from build123d import *
from build123d.topology import SkipClean

# Parameters (mm, degrees)
SKETCH2_R               = 70.00000000000001
BOSS_EXTRUDE1_DEPTH     = 500
SKETCH5_R               = 70.00000000000003
CUT_EXTRUDE1_DEPTH      = 500
CUT_EXTRUDE2_DEPTH      = 70
CUT_EXTRUDE2_DEPTH_BACK = 100
SKETCH6_W               = 70
SKETCH6_H               = 140
CUT_EXTRUDE3_DEPTH      = 120
CUT_EXTRUDE3_DEPTH_BACK = 100
SKETCH7_R               = 25
SKETCH8_R               = 25.000000000000007
CUT_EXTRUDE4_DEPTH      = 50


with BuildPart() as part:
    # Sketch2 → Boss-Extrude1 (new body)
    with BuildSketch(Plane(origin=(0, 0, 0), x_dir=(1, 0, 0), z_dir=(0, 1, 0))):
        with Locations(Location((0, 0, 0), (0, 0, 270))):
            Circle(SKETCH2_R)
    extrude(amount=BOSS_EXTRUDE1_DEPTH)

    # Sketch3 one side → Revolve1 (revolve)
    with SkipClean():  # the faces are left unmerged after this step: merging them gives an invalid solid
        with BuildSketch(Plane(origin=(0, 0, 0), x_dir=(-1, 0, 0), z_dir=(0, -1, 0))):
            with BuildLine():
                ThreePointArc((-1.505e-12, -70.00000000000001), (49.497474683057796, -49.49747468305888), (70.00000000000001, -2.07e-14))
                ThreePointArc((70.00000000000001, -3.55e-15), (49.497474683058854, 49.49747468305782), (1.46534e-12, 70.00000000000001))
                Line((0, 70.00000000000001), (0, -70.00000000000001))
            make_face()
        revolve(axis=Axis((0, 0, 0), (0, 0, 1)))

    # Sketch4 → Revolve2 (revolve)
    with SkipClean():  # the faces are left unmerged after this step: merging them gives an invalid solid
        with BuildSketch(Plane(origin=(0, 500, 0), x_dir=(1, 0, 0), z_dir=(0, 1, 0))):
            with BuildLine():
                Line((0, 70.00000000000001), (0, -70.00000000000001))
                ThreePointArc((0, -70.00000000000001), (70.00000000000001, 0), (0, 70.00000000000001))
            make_face()
        revolve(axis=Axis((0, 500, -70.00000000000001), (0, 0, 1)))

    # Sketch5 → Cut-Extrude1 (cut)
    with SkipClean():  # the faces are left unmerged after this step: merging them gives an invalid solid
        with BuildSketch(Plane(origin=(0, 0, 0), x_dir=(0, 0, -1), z_dir=(1, 0, 0))):
            with Locations((0, 500)):
                Circle(SKETCH5_R)
        extrude(amount=-CUT_EXTRUDE1_DEPTH, mode=Mode.SUBTRACT)

    # Sketch6 → Cut-Extrude2 (cut, two sides: drawn at the far end of the back side and taken through both)
    with BuildSketch(Plane(origin=(0, 0, 0), x_dir=(1, 0, 0), z_dir=(0, 1, 0)).offset(-CUT_EXTRUDE2_DEPTH_BACK)):
        Rectangle(SKETCH6_W, SKETCH6_H)
    extrude(amount=CUT_EXTRUDE2_DEPTH + CUT_EXTRUDE2_DEPTH_BACK, mode=Mode.SUBTRACT)

    # Sketch7 → Cut-Extrude3 (cut, two sides: drawn at the far end of the back side and taken through both)
    with BuildSketch(Plane.ZY.offset(-35).offset(-CUT_EXTRUDE3_DEPTH_BACK)):
        with Locations(Location((0, 0, 0), (0, 0, 180))):
            Circle(SKETCH7_R)
    extrude(amount=CUT_EXTRUDE3_DEPTH + CUT_EXTRUDE3_DEPTH_BACK, mode=Mode.SUBTRACT)

    # Sketch8 → Cut-Extrude4 (cut)
    with BuildSketch(Plane.ZY):
        with Locations((0, 500)):
            Circle(SKETCH8_R)
    extrude(amount=-CUT_EXTRUDE4_DEPTH, mode=Mode.SUBTRACT)


solid = part.part
For this review, take the finished solid that the model builds, in its own axes (mm). A direction names the side the tool comes from. Round coordinates to 2 decimals unless told otherwise and drop trailing zeros. Order: outer loops, then holes, each group sorted by start corner. A loop starts at its lowest first (then second) coordinate and runs counter-clockwise, first axis right, second up. Notation, with made-up numbers: M 12,88 L 71,88 A15 cw 71,117 Z; hole C -26.5,86.25 d9. An arc over 180 degrees is marked long. Write each question's results on one line, items separated by ' | '. Start each with the question number.
1. Clearance check with flat-ended pins moving along their axes: pin 1 Ø12 at (x, z) = (-17.5, -26.5) entering from -Y; pin 2 Ø5 at (x, z) = (52.5, -3.5) entering from -Y; pin 3 Ø1.5 at (x, y) = (43.5, 211.5) entering from +Z. State where each tip first meets the part, or that it passes through.
2. Add section B-B (x = 25). State the section outline as (y, z) points, then the cut area to 3 significant figures.
3. To check wall thickness, follow L1, parallel to Y at x = -57, z = 11.5; L2, parallel to X at y = 246, z = -4; L3, parallel to Z at x = 43, y = -10.5. State the ranges of each line that lie inside material, in increasing order. Write a range as [from, to].
4. Draft analysis for pull direction Z (two halves, no side actions). For faces 5 (the face through (35, 33, 1)), 6 (the face through (52.7, 22.2, -11.5)), 7 (the face through (69.404, 246.5, -9.113)), state which applies: pulls with the +Z half, pulls with the -Z half, needs draft (parallel to the pull), parting line crosses it, or undercut.
5. Add section A-A (z = 0). State the section outline as (x, y) points, then the cut area to 3 significant figures.
6. Tool access review of faces 1 (the face through (24.65, 524.787, -3.255)), 2 (the face through (-52.3, 22.2, -11.5)), 3 (the face through (-26.732, 430.017, 1.539)), 4 (the face through (0, 70, -1)): name each direction out of +Z, -Z, +X, -X, +Y, -Y from which nothing blocks a thin tool from reaching the whole face with its end or side.
7. Add section D-D (y = 104.5). State the section outline as (x, z) points, then the cut area to 3 significant figures.
8. Add section C-C (z = 36.5). State the section outline as (x, y) points.
Output values:
1) pin 1: y = 70 | pin 2: y = -48.87 | pin 3: z = 55.43
2) outline: M 70,-65.38 L 500,-65.38 A65.38 ccw 500,65.38 L 70,65.38 Z; hole C 500,0 d50 | area: 61,000 mm^2
3) L1: [-38.97, -22.2], [22.2, 430.95] | L2: [-69.89, 69.89] | L3: [-54.23, -22.69], [22.69, 54.23]
4) face 5: needs draft | face 6: undercut | face 7: parting line crosses it
5) outline: M -70,25 L -35,25 L -35,70 L 35,70 L 35,25 L 70,25 L 70,500 A70 ccw 0,570 L 0,525 L 50,525 L 50,475 L 0,475 L 0,430 L -70,430 Z; M -65.38,-25 A70 ccw -35,-60.62 L -35,-25 Z; M 35,-60.62 A70 ccw 65.38,-25 L 35,-25 Z | area: 61,100 mm^2
6) face 1: -X | face 2: +X, -X | face 3: -X, +Y | face 4: +Z, -Z, -Y
7) outline: C 0,0 d140 | area: 15,400 mm^2
8) outline: M -59.73,0 A59.73 ccw -35,-48.4 L -35,70 L 35,70 L 35,-48.4 A59.73 ccw 59.73,0 L 59.73,500 A59.73 ccw 0,559.73 L 0,440.27 L -59.73,440.27 Z
